Work out the finished part from the listing and answer in its coordinate system (mm). Face numbers are marked on the shaded views. A direction names the side the tool comes from. Round coordinates to 2 decimals unless told otherwise and drop trailing zeros. Order: outer loops, then holes, each group sorted by start corner. A loop starts at its lowest first (then second) coordinate and runs counter-clockwise, first axis right, second up. Notation, with made-up numbers: M 78.5,29.25 L 118.5,29.25 A20 ccw 118.5,63.25 Z; hole C 49,-10 d3. An arc over 180 degrees is marked long. Return JSON: item names as keys, results as strings.
from build123d import *

# Parameters (mm, degrees)
BOSS_EXTRUDE1_DEPTH = 30
CHAMFER1_SIZE       = 5
SKETCH2_R           = 3
CUT_EXTRUDE1_DEPTH  = 41


with BuildPart() as part:
    # Sketch1 → Boss-Extrude1 (new body, symmetric)
    with BuildSketch(Plane(origin=(0, 0, 0), x_dir=(1, 0, 0), z_dir=(0, 1, 0))):
        with BuildLine():
            Line((-60, 20), (-40, 20))
            ThreePointArc((-40, 20), (-20, 0), (-40, -20))
            Line((-40, -20), (-60, -20))
            ThreePointArc((-60, -20), (-80, 0), (-60, 20))
        make_face()
        with BuildLine():
            Line((-60, 10), (-40, 10))
            ThreePointArc((-40, 10), (-30, 0), (-40, -10))
            Line((-40, -10), (-60, -10))
            ThreePointArc((-60, -10), (-70, 0), (-60, 10))
        make_face(mode=Mode.SUBTRACT)
    extrude(amount=BOSS_EXTRUDE1_DEPTH, both=True)

    # Chamfer1
    chamfer1_edges = [part.edges().sort_by_distance(p)[0] for p in [
        (-20, 30, 0),
        (-50, 30, -20),
        (-80, 30, 0),
        (-50, 30, 20),
    ]]
    chamfer(chamfer1_edges, length=CHAMFER1_SIZE)

    # Sketch2 → Cut-Extrude1 (cut, through all)
    with BuildSketch(Plane.XY.offset(20)):
        with Locations((-50, 0.75)):
            Circle(SKETCH2_R)
    extrude(amount=-CUT_EXTRUDE1_DEPTH, mode=Mode.SUBTRACT)


solid = part.part
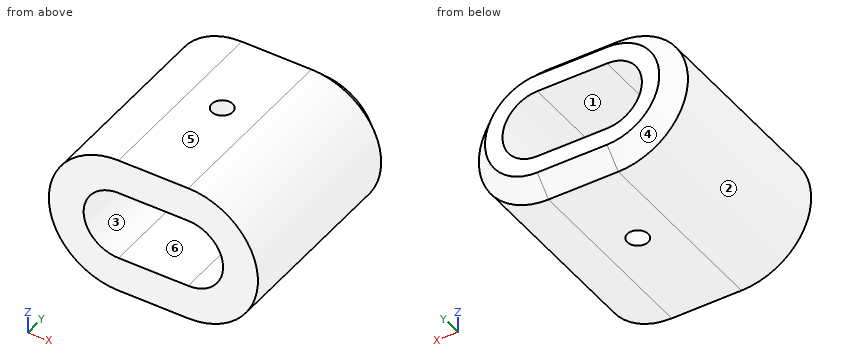
Item 1: The mould has two halves that part along X. Classify the marked faces 3, 4, 5 and 6: pulls with the +X half, pulls with the -X half, needs draft (parallel to the pull), parting line crosses it, or undercut.
Output:
{"face 3": "undercut", "face 4": "pulls with the -X half", "face 5": "needs draft", "face 6": "undercut"}
Item 2: Which of the six approach directions +Z, -Z, +X, -X, +Y, -Y give full straight-line access (tool end or side, diameter ignored) to the marked faces 1 and 2?
Output:
{"face 1": "+Y, -Y", "face 2": "-X, +Y, -Y"}
Item 3: Find section B-B (x = -50). Determine the outline of the cut face in (y, z).
Output:
{"outline": "M -30,-20 L -2.25,-20 L -2.25,-10 L -30,-10 Z; M -30,10 L -2.25,10 L -2.25,20 L -30,20 Z; M 3.75,-20 L 25,-20 L 30,-15 L 30,-10 L 3.75,-10 Z; M 3.75,10 L 30,10 L 30,15 L 25,20 L 3.75,20 Z"}
Item 4: Each of these flat-tipped pins is pushed along its axis until it touches: pin 1 (5 mm diameter, centred on x = -56.5, z = 6.5, fed in from -Y); pin 2 (1 mm diameter, centred on y = 7, z = -2, fed in from -X); pin 3 (2 mm diameter, centred on x = -33.5, y = 3, fed in from -Z). Where does it stop, or does it pass through?
Output:
{"pin 1": "passes through", "pin 2": "stops at x = -79.94", "pin 3": "stops at z = -19.23"}
Item 5: Consider line 1 along X through (y, z) = (-14.5, 0.5); line 2 along Y through (x, z) = (-50, 13); line 3 along Z through (x, y) = (-52.5, -8). Determine where each line is inside the solid, lowest interval first. Write a range as [from, to].
Output:
{"line 1": "x = [-79.99, -69.99], [-30.01, -20.01]", "line 2": "y = [-30, -2.25], [3.75, 30]", "line 3": "z = [-20, -10], [10, 20]"}
Item 6: Find section A-A (z = 0). Determine the outline of the cut face in (x, y), plus the area to 4 significant figures.
Output:
{"outline": "M -80,-30 L -70,-30 L -70,30 L -75,30 L -80,25 Z; M -30,-30 L -20,-30 L -20,25 L -25,30 L -30,30 Z", "area": "1,175 mm^2"}
